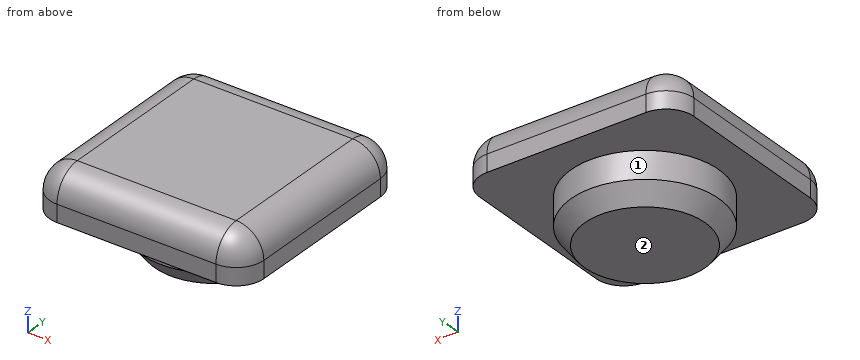
Autodesk Inventor part; units mm, degrees
ref_plane "CAP_XY" through (0, 0, 0) normal (0, 0, 1) x (1, 0, 0)
ref_plane "CAP_YZ" through (0, 0, 0) normal (1, 0, 0) x (0, 1, 0)
ref_plane "CAP_ZX" through (0, 0, 0) normal (0, 1, 0) x (0, 0, 1)
sketch "Sketch_4" plane through (0, 0, 0) normal (0, 1, 0) x (-1, 0, 0)
  arc A0 (7.75, -2) -> (5.75, 0) centre (5.75, -2) ccw
  line L0 (5.75, 0) -> (-5.75, 0)
  arc A1 (-5.75, 0) -> (-7.75, -2) centre (-5.75, -2) ccw
  line L1 (-7.75, -2) -> (-7.75, -3.25)
  line L2 (-7.75, -3.25) -> (7.75, -3.25)
  line L3 (7.75, -3.25) -> (7.75, -2)
extrude "Extrusion1" add sketch "Sketch_4" along normal mid plane 11.5
sketch "Sketch_5" plane through (0, 0, 0) normal (1, 0, 0) x (0, 1, 0)
  line L0 (5.75, 0) -> (-5.75, 0)
  arc A0 (-5.75, 0) -> (-7.75, -2) centre (-5.75, -2) ccw
  line L1 (-7.75, -2) -> (-7.75, -3.25)
  line L2 (-7.75, -3.25) -> (7.75, -3.25)
  line L3 (7.75, -3.25) -> (7.75, -2)
  arc A1 (7.75, -2) -> (5.75, 0) centre (5.75, -2) ccw
extrude "Extrusion2" add sketch "Sketch_5" along normal mid plane 11.5
sketch "Sketch_6" plane through (-5.75, 0, 0) normal (1, 0, 0) x (0, 0, -1)
  line L0 (3.25, 5.75) -> (0, 5.75)
  arc A0 (2, 7.75) -> (0, 5.75) centre (2, 5.75) ccw
  line L1 (2, 7.75) -> (3.25, 7.75)
  line L2 (3.25, 7.75) -> (3.25, 5.75)
  line L3 (3.25, 5.75) -> (0, 5.75)
revolve "Revolution1" add sketch "Sketch_6" angle 90 about axis through (-5.75, 5.75, -3.25) along (0, 0, 1)
sketch "Sketch_7" plane through (-5.75, 0, 0) normal (1, 0, 0) x (0, 0, -1)
  line L0 (0, -5.75) -> (3.25, -5.75)
  line L1 (3.25, -5.75) -> (3.25, -7.75)
  line L2 (3.25, -7.75) -> (2, -7.75)
  arc A0 (0, -5.75) -> (2, -7.75) centre (2, -5.75) ccw
  line L3 (0, -5.75) -> (3.25, -5.75)
revolve "Revolution2" add sketch "Sketch_7" angle 90 about axis through (-5.75, -5.75, 0) along (0, 0, -1)
sketch "Sketch_8" plane through (5.75, 0, 0) normal (1, 0, 0) x (0, 0, -1)
  line L0 (3.25, 5.75) -> (0, 5.75)
  arc A0 (2, 7.75) -> (0, 5.75) centre (2, 5.75) ccw
  line L1 (2, 7.75) -> (3.25, 7.75)
  line L2 (3.25, 7.75) -> (3.25, 5.75)
  line L3 (3.25, 5.75) -> (0, 5.75)
revolve "Revolution3" add sketch "Sketch_8" angle 90 about axis through (5.75, 5.75, -3.25) along (0, 0, -1)
sketch "Sketch_9" plane through (5.75, 0, 0) normal (1, 0, 0) x (0, 0, -1)
  line L0 (0, -5.75) -> (3.25, -5.75)
  line L1 (3.25, -5.75) -> (3.25, -7.75)
  line L2 (3.25, -7.75) -> (2, -7.75)
  arc A0 (0, -5.75) -> (2, -7.75) centre (2, -5.75) ccw
  line L3 (0, -5.75) -> (3.25, -5.75)
revolve "Revolution4" add sketch "Sketch_9" angle 90 about axis through (5.75, -5.75, 0) along (0, 0, 1)
sketch "Sketch_10" plane through (0, 0, 0) normal (0, 1, 0) x (-1, 0, 0)
  line L0 (0, 0) -> (0, -6.5)
  line L1 (0, -6.5) -> (-4.35, -6.5)
  line L2 (-4.35, -6.5) -> (-5.35, -5.2201)
  line L3 (-5.35, -5.2201) -> (-5.35, 0)
  line L4 (-5.35, 0) -> (0, 0)
  line L5 (0, 0) -> (0, -6.5)
revolve "Revolution5" add sketch "Sketch_10" angle 360 about axis through (0, 0, 0) along (0, 0, 1)
ref_plane "CAP_XY" through (0, 0, 0) normal (0, 0, 1) x (1, 0, 0)
ref_plane "CAP_YZ" through (0, 0, 0) normal (1, 0, 0) x (0, 1, 0)
ref_plane "CAP_ZX" through (0, 0, 0) normal (0, 1, 0) x (0, 0, 1)
properties part number "0000-00189079(1)"
Geometry: final body of the model. Coordinates: model frame, mm. Face numbers are marked on the shaded views. A direction names the side the tool comes from. Round coordinates to 2 decimals unless told otherwise and drop trailing zeros. Order: outer loops, then holes, each group sorted by start corner. A loop starts at its lowest first (then second) coordinate and runs counter-clockwise, first axis right, second up. Notation, with made-up numbers: (-14.5, 89.5) -> (1.5, 89.5) arc R30 cw to (1.5, 112.5) -> close; hole circle Ø6 at (17, -4). An arc over 180 degrees is marked (long way). Write each question's results on one line, items separated by ' | '.
Q1. Access query for the marked faces 1 and 2. Directions: +Z, -Z, +X, -X, +Y, -Y. A direction counts if a zero-diameter tool reaches every point of the face in a straight line with its end or side. Return the directions, or none.
Response values:
face 1: -Z | face 2: -Z, +X, -X, +Y, -Y
Q2. Section query A-A (x = 0). Output: boundary loops of the cut face in (y, z), and give its area (3 significant figures).
Response values:
outline: (-7.75, -3.25) -> (-5.35, -3.25) -> (-5.35, -5.22) -> (-4.35, -6.5) -> (4.35, -6.5) -> (5.35, -5.22) -> (5.35, -3.25) -> (7.75, -3.25) -> (7.75, -2) arc R2 ccw to (5.75, 0) -> (-5.75, 0) arc R2 ccw to (-7.75, -2) -> close | area: 82.2 mm²
Q3. Pin query (flat end, axial travel): pin 1 Ø1 at (x, y) = (-4.5, 6) entering from -Z; pin 2 Ø1.5 at (x, z) = (5.5, -5) entering from -Y. Return the tip coordinate at first contact, or that it passes through.
Response values:
pin 1: z = -3.25 | pin 2: y = -2.46
Q4. Section query C-C (z = -0.25). Output: boundary loops of the cut face in (x, y), and give its area (3 significant figures).
Response values:
outline: (-6.72, -5.75) arc R0.97 ccw to (-5.75, -6.72) -> (5.75, -6.72) arc R0.97 ccw to (6.72, -5.75) -> (6.72, 5.75) arc R0.97 ccw to (5.75, 6.72) -> (-5.75, 6.72) arc R0.97 ccw to (-6.72, 5.75) -> close | area: 180 mm²
Q5. Ray query, line 1 along Z through (x, y) = (-4.25, 4.5); line 2 along X through (y, z) = (4.5, -1.5); line 3 along Y through (x, z) = (-0.75, -0.75). Return the intervals inside material, ascending.
Response values:
line 1: -3.25 to 0 | line 2: -7.69 to 7.69 | line 3: -7.31 to 7.31
Q6. Section query D-D (z = -3.75). Output: boundary loops of the cut face in (x, y), and give its area (3 significant figures).
Response values:
outline: circle Ø10.7 at (0, 0) | area: 89.9 mm²
